Here's how the part is built. I have some questions about the finished solid (model axes, mm). A direction names the side the tool comes from. Coordinates: 2 decimals unless noted, no trailing zeros. Loops run counter-clockwise (first coordinate to the right, second up) from the corner with the lowest first, then second, coordinate; pieces in that order, holes last. Notation, with made-up numbers: (-39, 52) - (-3, 52) arc R7 ccw to (-3, 64) - close; hole circle Ø6 at (77.5, 60). An arc over 180 degrees is marked (long way). Use a Markdown table: item, result.
```python
from build123d import *

# Parameters (mm, degrees)
SZKIC1_W                    = 25.8
SZKIC1_H                    = 60
DODANIE_WYCI_GNI_CIE1_DEPTH = 4
OTW_R_POD_RUB_M21_D         = 2.6
ZAOKR_GLENIE1_R             = 2
WYTNIJ_WYCI_GNI_CIE1_REACH  = 6


with BuildPart() as part:
    # Szkic1 → Dodanie-wyciągnięcie1 (new body)
    with BuildSketch(Plane.XY):
        Rectangle(SZKIC1_W, SZKIC1_H)
    extrude(amount=DODANIE_WYCI_GNI_CIE1_DEPTH)

    # Otwór pod śrubę M21 (through all)
    with Locations(Plane.XY.offset(4)):
        with Locations((-10, 25), (10, 25), (10, -25), (-10, -25)):
            Hole(OTW_R_POD_RUB_M21_D / 2)

    # Zaokrąglenie1
    zaokr_glenie1_edges = [part.edges().sort_by_distance(p)[0] for p in [
        (12.9, -30, 2),
        (-12.9, -30, 2),
        (-12.9, 30, 2),
        (12.9, 30, 2),
    ]]
    fillet(zaokr_glenie1_edges, radius=ZAOKR_GLENIE1_R)

    # Szkic5 → Wytnij-wyciągnięcie1 (cut, up to next)
    with BuildSketch(Plane.XY.offset(4), mode=Mode.PRIVATE) as wytnij_wyci_gni_cie1_sk1:
        with BuildLine():
            Line((5, 20), (-5, 20))
            ThreePointArc((-5, 20), (-8.535533906, 18.535533906), (-10, 15))
            Line((-10, 15), (-10, -15))
            ThreePointArc((-10, -15), (-8.535533906, -18.535533906), (-5, -20))
            Line((-5, -20), (5, -20))
            ThreePointArc((5, -20), (8.535533906, -18.535533906), (10, -15))
            Line((10, -15), (10, 15))
            ThreePointArc((10, 15), (8.535533906, 18.535533906), (5, 20))
        make_face()
    wytnij_wyci_gni_cie1_tool1 = extrude(wytnij_wyci_gni_cie1_sk1.sketch, amount=-WYTNIJ_WYCI_GNI_CIE1_REACH, mode=Mode.PRIVATE) & part.part
    add(wytnij_wyci_gni_cie1_tool1.solids().sort_by_distance((0, 0, 4))[0], mode=Mode.SUBTRACT)


solid = part.part
```
Q1. I want a section at B-B, the plane y = -25. Write out the boundary of the cut face in (x, z).
Check values:
| item | result |
|---|---|
| outline | (-12.9, 0) - (-11.3, 0) - (-11.3, 4) - (-12.9, 4) - close; (-8.7, 0) - (8.7, 0) - (8.7, 4) - (-8.7, 4) - close; (11.3, 0) - (12.9, 0) - (12.9, 4) - (11.3, 4) - close |
Q2. I want a section at A-A, the plane z = 3.05. Write out the boundary of the cut face in (x, y), then the cut area to 3 significant figures.
Check values:
| item | result |
|---|---|
| outline | (-12.9, -28) arc R2 ccw to (-10.9, -30) - (10.9, -30) arc R2 ccw to (12.9, -28) - (12.9, 28) arc R2 ccw to (10.9, 30) - (-10.9, 30) arc R2 ccw to (-12.9, 28) - close; hole circle Ø2.6 at (-10, -25); hole circle Ø2.6 at (-10, 25); hole (-10, -15) arc R5 ccw to (-5, -20) - (5, -20) arc R5 ccw to (10, -15) - (10, 15) arc R5 ccw to (5, 20) - (-5, 20) arc R5 ccw to (-10, 15) - close; hole circle Ø2.6 at (10, -25); hole circle Ø2.6 at (10, 25) |
| area | 745 mm^2 |
Q3. If we mould it in two halves opening along X, with no side actions, what happens to faces 3 (the face through (10, 0, 2)), 4 (the face through (-10.6, 23.847, 1.972)), 5 (the face through (-12.9, 0, 2)), 6 (the face through (12.9, 0, 2))? For each: pulls with the +X half, pulls with the -X half, needs draft (parallel to the pull), parting line crosses it, or undercut.
Check values:
| item | result |
|---|---|
| face 3 | undercut |
| face 4 | undercut |
| face 5 | pulls with the -X half |
| face 6 | pulls with the +X half |
Q4. Please list where these lines run through material, in increasing order: L1, parallel to Y at x = 2.5, z = 2.5; L2, parallel to Y at x = -9.5, z = 3.5; L3, parallel to X at y = 14, z = 3.2. Write a range as from..to.
Check values:
| item | result |
|---|---|
| L1 | -30..-20, 20..30 |
| L2 | -30..-26.2, -23.8..-17.18, 17.18..23.8, 26.2..30 |
| L3 | -12.9..-10, 10..12.9 |
Q5. I want a section at C-C, the plane x = 3. Write out the boundary of the cut face in (y, z), then the cut area to 3 significant figures.
Check values:
| item | result |
|---|---|
| outline | (-30, 0) - (-20, 0) - (-20, 4) - (-30, 4) - close; (20, 0) - (30, 0) - (30, 4) - (20, 4) - close |
| area | 80.0 mm^2 |
Q6. I want a section at D-D, the plane y = 7.5. Write out the boundary of the cut face in (x, z).
Check values:
| item | result |
|---|---|
| outline | (-12.9, 0) - (-10, 0) - (-10, 4) - (-12.9, 4) - close; (10, 0) - (12.9, 0) - (12.9, 4) - (10, 4) - close |
Q7. Which directions (+Z, -Z, +X, -X, +Y, -Y) give clear straight access to the entire face, cutting with the end or side of a thin tool? Please do faces 1 (the face through (12.3, -29.43, 2.03)), 2 (the face through (-8, 19, 2)).
Check values:
| item | result |
|---|---|
| face 1 | +Z, -Z, +X, -Y |
| face 2 | +Z, -Z |
